```python
from build123d import *

# Parameters (mm, degrees)
SKETCH1_R           = 3.2639
BOSS_EXTRUDE1_DEPTH = 1.5875


with BuildPart() as part:
    # Sketch1 → Boss-Extrude1 (new body, symmetric)
    with BuildSketch(Plane(origin=(0, 0, 0), x_dir=(0, 0, -1), z_dir=(1, 0, 0))):
        with BuildLine():
            Line((-38.1, 9.525), (-38.1, -9.525))
            Line((-38.1, -9.525), (-0.02243898, -9.613873814))
            ThreePointArc((-0.02243898, -9.613873814), (9.6139, 0), (-0.02243898, 9.613873814))
            Line((-0.02243898, 9.613873814), (-38.1, 9.525))
        make_face()
        Circle(SKETCH1_R, mode=Mode.SUBTRACT)
    extrude(amount=BOSS_EXTRUDE1_DEPTH, both=True)


solid = part.part
```
Can you work these out from the model? Positions are in its coordinate system, mm. Coordinates: 2 decimals unless noted, no trailing zeros. Write each loop counter-clockwise with the first axis right and the second up, starting at its lowest first coordinate (ties: lowest second). Pieces come first, ordered by that corner, then holes. Notation, with made-up numbers: M 45,89 L 83,89 A26 cw 83,112 Z; hole C 88,31 d9. An arc over 180 degrees is marked long. Write item = value, one per line. Start each with the question number.
Q1. If we section it at B-B, the plane z = -1.5: Write out the boundary of the cut face in (x, y), then the cut area to 3 significant figures.
Q2. Thinking about a two-plate mould opening in Y: for faces 1 (the face through (0.02, -0.21, -9.61)), 2 (the face through (1.588, 0, 15)), 3 (the face through (-0.022, -3.186, 0.708)), which applies, released by +Y, released by -Y, zero draft, split by the parting line, or undercut?
Q3. If we section it at D-D, the plane y = -7.25: Write out the boundary of the cut face in (x, z), then the cut area to 3 significant figures.
Q4. If we section it at C-C, the plane x = -1.05: Write out the boundary of the cut face in (y, z) (3 decimals).
Q5. If we section it at A-A, the plane y = 0: Write out the boundary of the cut face in (x, z), then the cut area to 3 significant figures.
Q6. If I drill on L1, parallel to Y at x = 0.5, z = 0; L2, parallel to Y at x = 0.5, z = 3.5; L3, parallel to Y at x = 0.4, z = 3, over which ranges is the centre line in solid material (lowest first)? Write a range as [from, to].
Q7. I'm going to push a flat-ended pin straight in: pin 1 (1 mm diameter, centred on x = 0.5, z = 26.5, fed in from -Y). Where does the tip first touch, or does it pass through?
Check sheet entries:
q1.outline = M -1.59,-9.5 L 1.59,-9.5 L 1.59,-2.9 L -1.59,-2.9 Z; M -1.59,2.9 L 1.59,2.9 L 1.59,9.5 L -1.59,9.5 Z
q1.area = 41.9 mm²
q2.face_1 = split by the parting line
q2.face_2 = zero draft
q2.face_3 = undercut
q3.outline = M -1.59,-6.31 L 1.59,-6.31 L 1.59,38.1 L -1.59,38.1 Z
q3.area = 141 mm²
q4.outline = M -9.614,0.022 A9.614 ccw 9.614,0.022 L 9.525,38.1 L -9.525,38.1 Z; hole C 0,0 d6.528
q5.outline = M -1.59,-9.61 L 1.59,-9.61 L 1.59,-3.26 L -1.59,-3.26 Z; M -1.59,3.26 L 1.59,3.26 L 1.59,38.1 L -1.59,38.1 Z
q5.area = 131 mm²
q6.L1 = [-9.61, -3.26], [3.26, 9.61]
q6.L2 = [-9.61, 9.61]
q6.L3 = [-9.61, -1.29], [1.29, 9.61]
q7.pin_1 = -9.55
